Check sheet for the drawn part. Datum: minimum x, y, z corner. Units: mm. A direction names the side the tool comes from. Coordinates: 2 decimals unless noted, no trailing zeros. Order: outer loops, then holes, each group sorted by start corner. A loop starts at its lowest first (then second) coordinate and runs counter-clockwise, first axis right, second up. Notation, with made-up numbers: (-7.5, -34.5) - (36.5, -34.5) arc R23 cw to (36.5, -7.5) - close; hole circle Ø6 at (62.5, 47). An arc over 180 degrees is marked (long way). Return JSON: item names as keys, results as strings. Group by question number.
Item 1: Section check A-A on x = 3. Enter the section's corners in (y, z).
Item 2: Gauge pin test, flat ends, axial feed: pin 1 (1.5 mm diameter, centred on y = 10, z = 34.5, fed in from +X); pin 2 (2 mm diameter, centred on x = 117, z = 38.5, fed in from +Y); pin 3 (4 mm diameter, centred on x = 117, z = 3.5, fed in from +Y); pin 4 (7 mm diameter, centred on y = 6, z = 15.5, fed in from -X). Record the tip position at first contact, or that the pin passes through.
Item 3: Section check D-D on y = 4. Enter the section's corners in (x, z), then the cut area to 3 significant figures.
Item 4: Scan lines: probe 1 along X at (y, z) = (1.4, 38.5); probe 2 along Z at (x, y) = (3, 1.45); probe 3 along X at (y, z) = (11.75, 27). Record each from-to range of solid material in increasing order.
Item 5: Section check C-C on z = 16. Enter the section's corners in (x, y), then the cut area to 3 significant figures.
Item 6: Section check B-B on z = 21. Enter the section's corners in (x, y).
Item 7: Tool access check on the marked faces 1, 2 and 3. Record the directions out of +Z, -Z, +X, -X, +Y, -Y that give a thin tool (end or side, any length) a straight path to the whole face; none if there is none.
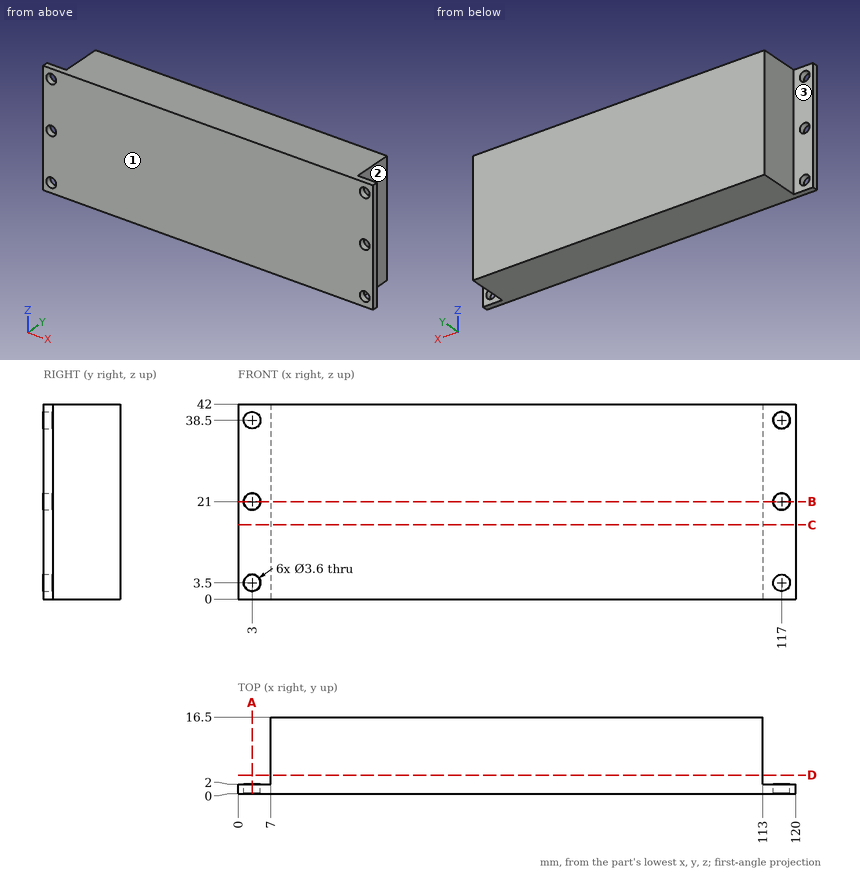
Computed:
{
 "1": {"outline": "(0, 0) - (2, 0) - (2, 1.7) - (0, 1.7) - close; (0, 5.3) - (2, 5.3) - (2, 19.2) - (0, 19.2) - close; (0, 22.8) - (2, 22.8) - (2, 36.7) - (0, 36.7) - close; (0, 40.3) - (2, 40.3) - (2, 42) - (0, 42) - close"},
 "2": {"pin 1": "stops at x = 113", "pin 2": "passes through", "pin 3": "stops at y = 2", "pin 4": "stops at x = 7"},
 "3": {"outline": "(7, 0) - (113, 0) - (113, 42) - (7, 42) - close", "area": "4,450 mm²"},
 "4": {"probe 1": "x = 0 to 1.2, 4.8 to 115.2, 118.8 to 120", "probe 2": "z = 0 to 1.7, 5.3 to 19.2, 22.8 to 36.7, 40.3 to 42", "probe 3": "x = 7 to 113"},
 "5": {"outline": "(0, 0) - (120, 0) - (120, 2) - (113, 2) - (113, 16.5) - (7, 16.5) - (7, 2) - (0, 2) - close", "area": "1,780 mm²"},
 "6": {"outline": "(0, 0) - (1.2, 0) - (1.2, 2) - (0, 2) - close; (4.8, 0) - (115.2, 0) - (115.2, 2) - (113, 2) - (113, 16.5) - (7, 16.5) - (7, 2) - (4.8, 2) - close; (118.8, 0) - (120, 0) - (120, 2) - (118.8, 2) - close"},
 "7": {"face 1": "+Z, -Z, +X, -X, -Y", "face 2": "+Z, -Z, +X, +Y", "face 3": "+Z, -Z, -X, +Y"}
}
